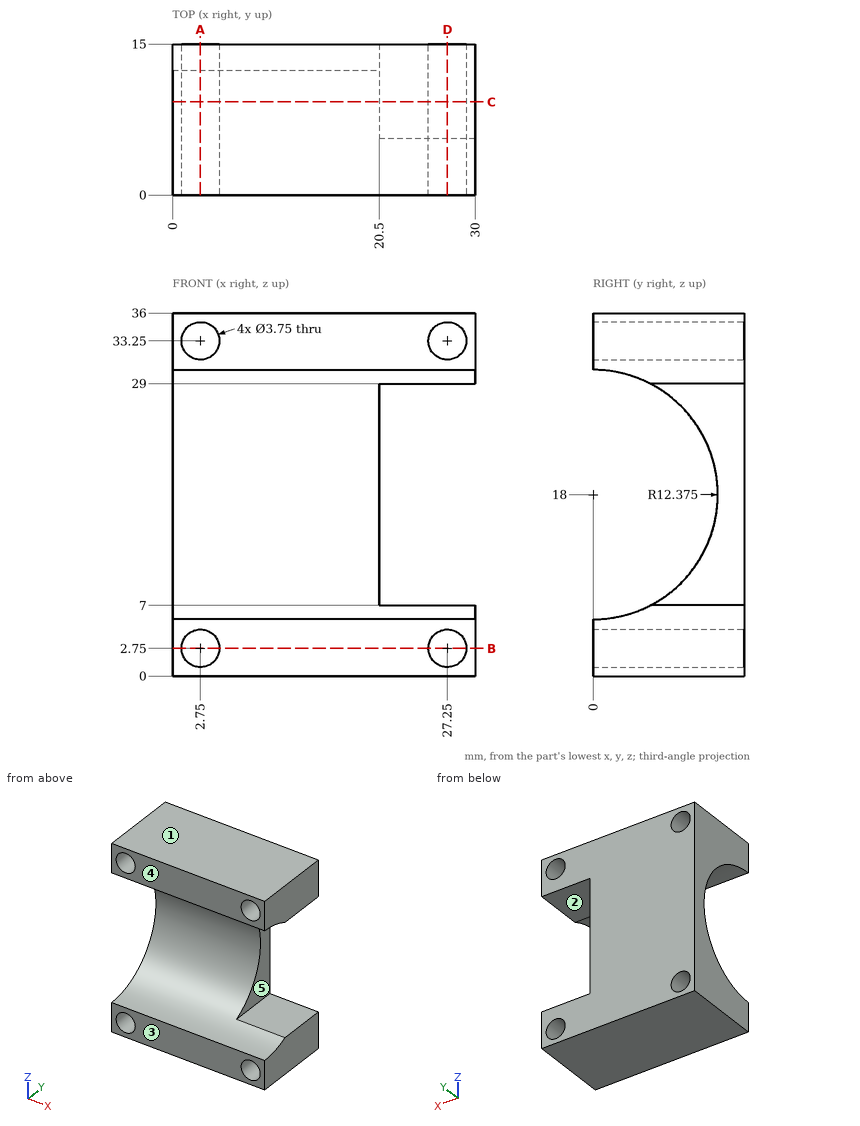
Study the drawing (mm; zero at the part's minimum x, y, z) and answer. A direction names the side the tool comes from. Give positions to 0.01 mm unless a question says otherwise; leave off trailing zeros. Loops run counter-clockwise (first coordinate to the right, second up) from the corner with the lowest first, then second, coordinate; pieces in that order, holes last. Notation, with made-up numbers: M 83.25,89 L 139.25,89 A28 ccw 139.25,126 Z; hole C 45.25,13 d3. An arc over 180 degrees is marked long. One line per item, written item: value.
1. Section C-C on y = 9.25 is taken. Determine the outline of the cut face in (x, z) (3 decimals).
Found:
outline: M 0,0 L 30,0 L 30,7 L 20.5,7 L 20.5,9.779 L 0,9.779 Z; M 0,26.221 L 20.5,26.221 L 20.5,29 L 30,29 L 30,36 L 0,36 Z; hole C 2.75,2.75 d3.75; hole C 2.75,33.25 d3.75; hole C 27.25,2.75 d3.75; hole C 27.25,33.25 d3.75
2. For a pull along Z with two mould halves and no side action, classify the marked faces 1, 2 and 3 as pulls with the +Z half, pulls with the -Z half, needs draft (parallel to the pull), parting line crosses it, or undercut.
Found:
face 1: pulls with the +Z half
face 2: undercut
face 3: needs draft
3. Section D-D on x = 27.25 is taken. Determine the outline of the cut face in (y, z) (3 decimals), plus the area to 3 significant figures.
Found:
outline: M 0,0 L 15,0 L 15,0.875 L 0,0.875 Z; M 0,4.625 L 15,4.625 L 15,7 L 5.669,7 A12.375 cw 0,5.625 Z; M 0,30.375 A12.375 cw 5.669,29 L 15,29 L 15,31.375 L 0,31.375 Z; M 0,35.125 L 15,35.125 L 15,36 L 0,36 Z
area: 87.0 mm^2
4. Each of these flat-tipped pins is pushed along its axis until it touches: P1, Ø3.5, axis at x = 27.25, z = 33.25, coming from the -Y side (1 decimal); P2, Ø5, axis at y = 8.5, z = 24, coming from the +X side. Where does it stop, or does it pass through?
Found:
P1: through
P2: x = 20.5
5. Section A-A on x = 2.75 is taken. Determine the outline of the cut face in (y, z) (3 decimals).
Found:
outline: M 0,0 L 15,0 L 15,0.875 L 0,0.875 Z; M 0,4.625 L 15,4.625 L 15,31.375 L 0,31.375 L 0,30.375 A12.375 cw 0,5.625 Z; M 0,35.125 L 15,35.125 L 15,36 L 0,36 Z
6. Section B-B on z = 2.75 is taken. Determine the outline of the cut face in (x, y) (3 decimals), plus the area to 4 significant figures.
Found:
outline: M 0,0 L 0.875,0 L 0.875,15 L 0,15 Z; M 4.625,0 L 25.375,0 L 25.375,15 L 4.625,15 Z; M 29.125,0 L 30,0 L 30,15 L 29.125,15 Z
area: 337.5 mm^2
7. For the marked faces 4 and 5, determine the directions among +Z, -Z, +X, -X, +Y, -Y from which every point of the face is accessible in a straight line to the end or side of a thin tool.
Found:
face 4: +Z, -Z, +X, -X, -Y
face 5: +X, +Y, -Y
8. Find the intervals of material crossed by probe 1 along X at (y, z) = (9.5, 2.75) (3 decimals); probe 2 along Z at (x, y) = (27.25, 9) (3 decimals); probe 3 along Z at (x, y) = (2.75, 8.75) (3 decimals), in increasing order.
Found:
probe 1: 0 to 0.875, 4.625 to 25.375, 29.125 to 30
probe 2: 0 to 0.875, 4.625 to 7, 29 to 31.375, 35.125 to 36
probe 3: 0 to 0.875, 4.625 to 9.249, 26.751 to 31.375, 35.125 to 36
